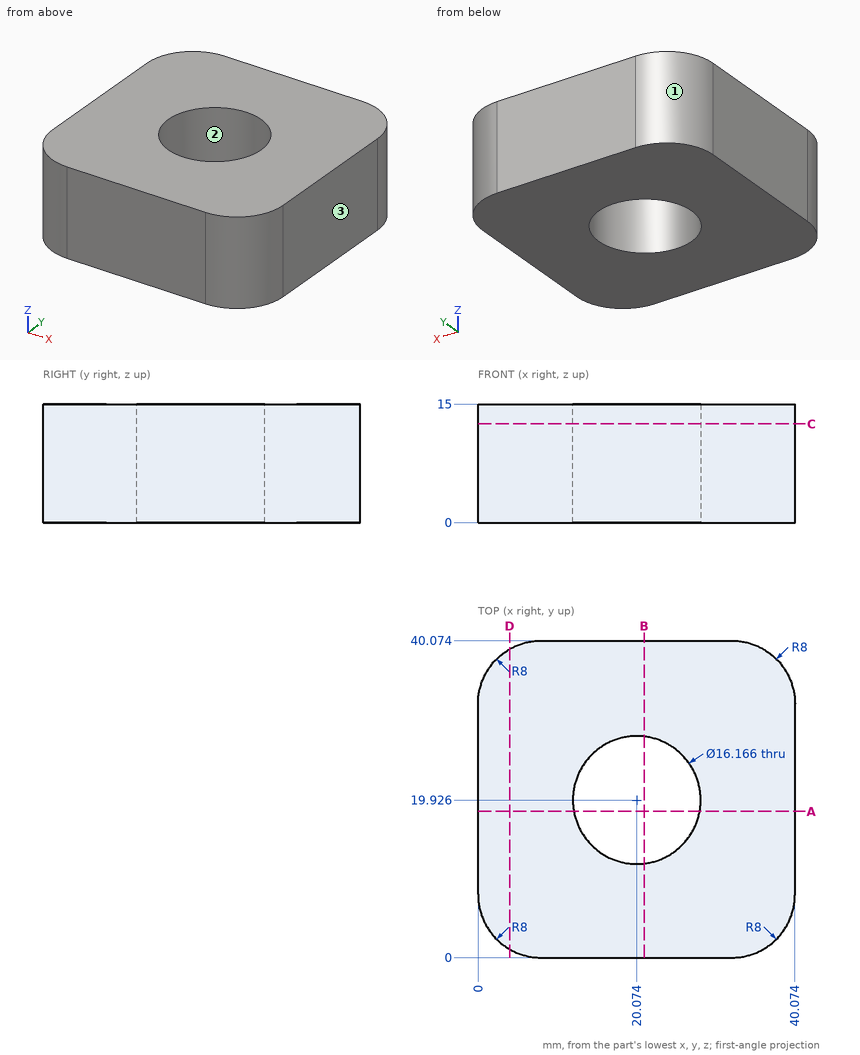
Verification items for this drawing (mm, ordinates from the low corner). Give positions to 0.01 mm unless a question says otherwise; leave off trailing zeros. Write each loop counter-clockwise with the first axis right and the second up, starting at its lowest first coordinate (ties: lowest second). Pieces come first, ordered by that corner, then holes. Notation, with made-up numbers: (17.5, -38) -> (56.5, -38) arc R15 ccw to (56.5, -23) -> close; hole circle Ø7 at (35, 52). An arc over 180 degrees is marked (long way). Write item = value, one per line.
Item 1: Sectioned sample at C-C on z = 12.5. Record the boundary of the cut face in (x, y) (1 decimal).
Output:
outline = (0, 8) arc R8 ccw to (8, 0) -> (32.1, 0) arc R8 ccw to (40.1, 8) -> (40.1, 32.1) arc R8 ccw to (32.1, 40.1) -> (8, 40.1) arc R8 ccw to (0, 32.1) -> close; hole circle Ø16.2 at (20.1, 19.9)
Item 2: Sectioned sample at A-A on y = 18.5. Record the boundary of the cut face in (x, z) (1 decimal).
Output:
outline = (0, 0) -> (12.1, 0) -> (12.1, 15) -> (0, 15) -> close; (28, 0) -> (40.1, 0) -> (40.1, 15) -> (28, 15) -> close
Item 3: Sectioned sample at B-B on x = 21. Record the boundary of the cut face in (y, z) (1 decimal), and give its area (3 significant figures).
Output:
outline = (0, 0) -> (11.9, 0) -> (11.9, 15) -> (0, 15) -> close; (28, 0) -> (40.1, 0) -> (40.1, 15) -> (28, 15) -> close
area = 360 mm^2
Item 4: Release check for a two-part mould opening along X. For the marked faces 1, 2 and 3 record: +X half, -X half, draft (parallel to the pull), parting line (faces both ways), or undercut.
Output:
face_1 = -X half
face_2 = undercut
face_3 = +X half
Item 5: Scan lines: probe 1 along X at (y, z) = (20, 4) (1 decimal); probe 2 along X at (y, z) = (24, 3.5) (1 decimal); probe 3 along Y at (x, z) = (18, 6.5) (1 decimal). Record each from-to range of solid material in increasing order. Write a range as from..to.
Output:
probe_1 = 0..12, 28.2..40.1
probe_2 = 0..13.1, 27.1..40.1
probe_3 = 0..12.1, 27.7..40.1
Item 6: Sectioned sample at D-D on x = 4. Record the boundary of the cut face in (y, z), and give its area (3 significant figures).
Output:
outline = (1.07, 0) -> (39, 0) -> (39, 15) -> (1.07, 15) -> close
area = 569 mm^2
Item 7: Gauge pin test, flat ends, axial feed: pin 1 (2 mm diameter, centred on y = 6, z = 11, fed in from -X); pin 2 (1 mm diameter, centred on y = 6.5, z = 3.5, fed in from +X); pin 3 (4 mm diameter, centred on y = 36, z = 6.5, fed in from -X) (1 decimal). Record the tip position at first contact, or that the pin passes through.
Output:
pin_1 = 0.06
pin_2 = 40.01
pin_3 = 0.2
